from build123d import *

# Parameters (mm, degrees)
DODANIE_WYCI_GNI_CIE1_DEPTH = 15


with BuildPart() as part:
    # Szkic1 → Dodanie-wyciągnięcie1 (new body)
    with BuildSketch(Plane.XY):
        with BuildLine():
            Line((-11.5, 0), (-29, 0))
            Line((-29, 0), (-29, -16.5))
            Line((-29, -16.5), (29, -16.5))
            Line((29, -16.5), (29, 0))
            Line((29, 0), (11.5, 0))
            ThreePointArc((11.5, 0), (0, -11.5), (-11.5, 0))
        make_face()
    extrude(amount=DODANIE_WYCI_GNI_CIE1_DEPTH)

    # Szkic3 → Otwory ustalające Ø6.0mm1 (revolve, cut)
    with BuildSketch(Plane(origin=(-23.5, 0, 7.5), x_dir=(0, 0, 1), z_dir=(1, 0, 0))):
        Polygon((0, 0), (0, 11.802581857), (3, 10), (3, 0), align=None)
    otwory_ustalaj_ce_6_0mm1 = revolve(axis=Axis((-23.5, 6.35, 7.5), (0, -1, 0)), mode=Mode.SUBTRACT)

    # Lustro1: Otwory ustalające Ø6.0mm1 across plane
    add(otwory_ustalaj_ce_6_0mm1.mirror(Plane(origin=(0, 0, 0), x_dir=(0, 0, 1), z_dir=(1, 0, 0))), mode=Mode.SUBTRACT)


solid = part.part
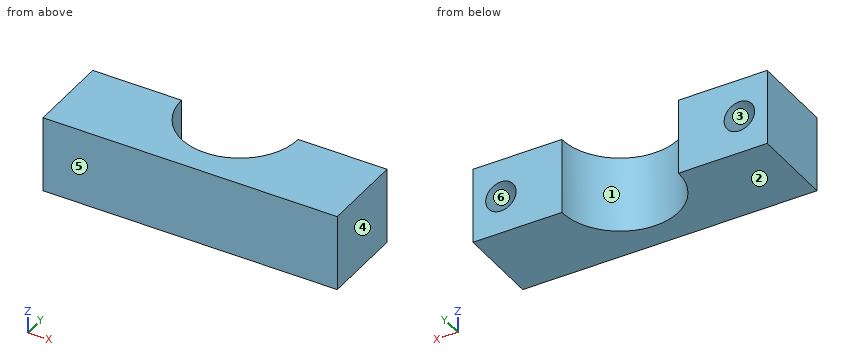
For this review, take the finished solid that the model builds, in its own axes (mm). Face numbers are marked on the shaded views. A direction names the side the tool comes from. Round coordinates to 2 decimals unless told otherwise and drop trailing zeros. Order: outer loops, then holes, each group sorted by start corner. A loop starts at its lowest first (then second) coordinate and runs counter-clockwise, first axis right, second up. Notation, with made-up numbers: M 70,-17 L 92,-17 A24 cw 92,-2 Z; hole C 54,46 d1. An arc over 180 degrees is marked long. Write each question's results on one line, items separated by ' | '. Start each with the question number.
1. To check wall thickness, follow L1, parallel to X at y = -2.75, z = 9.25; L2, parallel to X at y = -2, z = 4.75; L3, parallel to Z at x = -23.5, y = -2.5. State the ranges of each line that lie inside material, in increasing order. Write a range as [from, to].
2. Add section B-B (x = 0). State the section outline as (y, z) points.
3. Add section A-A (y = -9.5). State the section outline as (x, z) points, then the cut area to 3 significant figures.
4. Tool access review of the marked faces 5 and 6: name each direction out of +Z, -Z, +X, -X, +Y, -Y from which nothing blocks a thin tool from reaching the whole face with its end or side.
5. Add section C-C (z = 13.25). State the section outline as (x, y) points.
6. Add section D-D (y = -3). State the section outline as (x, z) points.
7. Clearance check with flat-ended pins moving along their axes: pin 1 Ø2 at (x, z) = (-4, 7.5) entering from +Y; pin 2 Ø3.5 at (x, z) = (-23.5, 7.5) entering from +Y. State where each tip first meets the part, or that it passes through.
8. Draft analysis for pull direction X (two halves, no side actions). For the marked faces 1, 2, 3 and 4, state which applies: pulls with the +X half, pulls with the -X half, needs draft (parallel to the pull), parting line crosses it, or undercut.
Output values:
1) L1: [-29, -25.94], [-21.06, -11.17], [11.17, 21.06], [25.94, 29] | L2: [-29, -24.7], [-22.3, -11.32], [11.32, 22.3], [24.7, 29] | L3: [0, 4.5], [10.5, 15]
2) outline: M -16.5,0 L -11.5,0 L -11.5,15 L -16.5,15 Z
3) outline: M -29,0 L -6.48,0 L -6.48,15 L -29,15 Z; M 6.48,0 L 29,0 L 29,15 L 6.48,15 Z; hole C -23.5,7.5 d6; hole C 23.5,7.5 d6 | area: 619 mm^2
4) face 5: +Z, -Z, +X, -X, -Y | face 6: +Y
5) outline: M -29,-16.5 L 29,-16.5 L 29,0 L 11.5,0 A11.5 cw -11.5,0 L -29,0 Z
6) outline: M -29,0 L -11.1,0 L -11.1,15 L -29,15 Z; M 11.1,0 L 29,0 L 29,15 L 11.1,15 Z; hole C -23.5,7.5 d6; hole C 23.5,7.5 d6
7) pin 1: y = -10.36 | pin 2: y = -10.75
8) face 1: undercut | face 2: needs draft | face 3: undercut | face 4: pulls with the +X half
